Autodesk Inventor part; units mm, degrees
ref_plane "YZ Plane" through (0, 0, 0) normal (1, 0, 0) x (0, 1, 0)
ref_plane "XZ Plane" through (0, 0, 0) normal (0, 1, 0) x (-1, 0, 0)
ref_plane "XY Plane" through (0, 0, 0) normal (0, 0, 1) x (1, 0, 0)
sketch "Sketch1" plane through (0, 0, 0) normal (0, 0, 1) x (1, 0, 0)
  line L0 (-20, 10) -> (20, 10)
  line L1 (20, 10) -> (20, -10)
  line L2 (20, -10) -> (-20, -10)
  line L3 (-20, -10) -> (-20, 10)
  line L4 (-20, 10) -> (20, -10) construction
  line L5 (20, 10) -> (-20, -10) construction
  line L6 (18, 8) -> (-18, 8)
  line L7 (-18, 8) -> (-18, -8)
  line L8 (-18, -8) -> (18, -8)
  line L9 (18, -8) -> (18, 8)
  point P0 (0, 0)
  dimension "d0" = 40
  dimension "d1" = 20
  dimension "d2" = 2
extrude "Extrusion1" add sketch "Sketch1" along normal mid plane 300
fillet "Fillet1" radius 2 4 edges at (-20, 10, 0) (-20, -10, 0) (20, -10, 0) (20, 10, 0)
properties part number "Leg tube 1"
Build history of the part. All positions in model axes, mm. A direction names the side the tool comes from. Give positions to 0.01 mm unless a question says otherwise; leave off trailing zeros. Loops run counter-clockwise (first coordinate to the right, second up) from the corner with the lowest first, then second, coordinate; pieces in that order, holes last.
Item 1: Slice it at B-B, the plane x = -3.5. List the corners of the cut face in (y, z), and give its area (3 significant figures).
Answers follow:
outline: (-10, -150) - (-8, -150) - (-8, 150) - (-10, 150) - close; (8, -150) - (10, -150) - (10, 150) - (8, 150) - close
area: 1,200 mm2
Item 2: Drill centre lines: line 1 (Y direction, x = 12, z = 58.5); line 2 (X direction, y = -6.75, z = -37); line 3 (X direction, y = -8.5, z = 18). Where is each one in solid material? Low to high.
Answers follow:
line 1: y = -10 to -8, 8 to 10
line 2: x = -20 to -18, 18 to 20
line 3: x = -19.94 to 19.94
Item 3: Which spindle directions (+Z, -Z, +X, -X, +Y, -Y) get a long thin tool onto all of the face, cutting with end or side? Do faces 1 (the face through (0, 10, -2)), 2 (the face through (-18, 0, -2)). Say none if no direction does.
Answers follow:
face 1: +Z, -Z, +X, -X, +Y
face 2: +Z, -Z
Item 4: Pull direction X, two halves, no side cores. Call faces 3 (the face through (0, -10, -2)), 4 (the face through (20, 0, -2)), 5 (the face through (0, 8, -2)), 6 (the face through (-20, 0, -2)): released by +X, released by -X, zero draft, split by the parting line, or undercut.
Answers follow:
face 3: zero draft
face 4: released by +X
face 5: undercut
face 6: released by -X
Item 5: Slice it at C-C, the plane y = -5.25. List the corners of the cut face in (x, z).
Answers follow:
outline: (-20, -150) - (-18, -150) - (-18, 150) - (-20, 150) - close; (18, -150) - (20, -150) - (20, 150) - (18, 150) - close
Item 6: Slice it at A-A, the plane z = -82. List the corners of the cut face in (x, y), and give its area (3 significant figures).
Answers follow:
outline: (-20, -8) arc R2 ccw to (-18, -10) - (18, -10) arc R2 ccw to (20, -8) - (20, 8) arc R2 ccw to (18, 10) - (-18, 10) arc R2 ccw to (-20, 8) - close; hole (-18, -8) - (18, -8) - (18, 8) - (-18, 8) - close
area: 221 mm2
